Check sheet for the modelled part. Datum: model origin and axes. Units: mm. A direction names the side the tool comes from. Coordinates: 2 decimals unless noted, no trailing zeros. Loops run counter-clockwise (first coordinate to the right, second up) from the corner with the lowest first, then second, coordinate; pieces in that order, holes last.
from build123d import *

# Parameters (mm, degrees)
SKETCH1_W           = 25.4
SKETCH1_H           = 25.4
BOSS_EXTRUDE1_DEPTH = 5.91
BOSS_EXTRUDE2_DEPTH = 25.4
BOSS_EXTRUDE3_DEPTH = 25.4
BOSS_EXTRUDE4_DEPTH = 25.4
FILLET2_R           = 1


with BuildPart() as part:
    # Sketch1 → Boss-Extrude1 (new body)
    with BuildSketch(Plane(origin=(0, 0, 0), x_dir=(1, 0, 0), z_dir=(0, 1, 0))):
        Rectangle(SKETCH1_W, SKETCH1_H)
    extrude(amount=BOSS_EXTRUDE1_DEPTH)

    # Sketch2 → Boss-Extrude2 (add)
    with BuildSketch(Plane.XY.offset(12.7)):
        Polygon((-3, 0), (3, 0), (3, 2.5), (6, 2.5), (6, 4.5), (4.585786438, 5.914213562), (-4.585786438, 5.914213562), (-6, 4.5), (-6, 2.5), (-3, 2.5), align=None)
    extrude(amount=BOSS_EXTRUDE2_DEPTH)

    # Sketch3 → Boss-Extrude3 (add)
    with BuildSketch(Plane.ZY.offset(12.7)):
        Polygon((-3, 0), (3, 0), (3, 2.5), (6, 2.5), (6, 4.5), (4.585786438, 5.914213562), (-4.585786438, 5.914213562), (-6, 4.5), (-6, 2.5), (-3, 2.5), align=None)
    extrude(amount=BOSS_EXTRUDE3_DEPTH)

    # Sketch5 → Boss-Extrude4 (add)
    with BuildSketch(Plane(origin=(0, 5.91, 0), x_dir=(1, 0, 0), z_dir=(0, 1, 0))):
        Polygon((3, 12.7), (-3, 12.7), (-3, 10.2), (-6, 10.2), (-6, 8.2), (-4.585786438, 6.785786438), (4.585786438, 6.785786438), (6, 8.2), (6, 10.2), (3, 10.2), align=None)
        Polygon((12.7, -3), (12.7, 3), (10.2, 3), (10.2, 6), (8.2, 6), (6.785786438, 4.585786438), (6.785786438, -4.585786438), (8.2, -6), (10.2, -6), (10.2, -3), align=None)
    extrude(amount=BOSS_EXTRUDE4_DEPTH)

    # Fillet2
    fillet2_edges = [part.edges().sort_by_distance(p)[0] for p in [
        (6.785786438, 5.91, 0),
        (7.492893219, 5.91, 5.292893219),
        (9.2, 5.91, 6),
        (10.2, 5.91, 4.5),
        (11.45, 5.91, 3),
        (12.7, 18.61, 3),
        (-12.7, 5.91, -8.645),
        (7.85, 0, 12.7),
        (8.645, 5.91, 12.7),
        (-8.645, 5.91, 12.7),
        (3, 0, 25.4),
        (-3, 0, 25.4),
        (0, 0, 38.1),
        (-12.7, 0, 7.85),
        (-12.7, 5.91, 8.645),
        (-25.4, 0, 3),
        (12.7, 5.91, 7.85),
        (-7.85, 0, 12.7),
        (-12.7, 0, -7.85),
        (-25.4, 0, -3),
        (-38.1, 0, 0),
        (0, 0, -12.7),
        (12.7, 0, 0),
        (12.7, 5.91, -7.85),
        (-7.85, 5.91, -12.7),
        (-3, 5.91, -11.45),
        (-3, 18.61, -12.7),
        (-4.5, 5.91, -10.2),
        (-6, 5.91, -9.2),
        (-5.292893219, 5.91, -7.492893219),
        (0, 5.91, -6.785786438),
        (5.292893219, 5.91, -7.492893219),
        (6, 5.91, -9.2),
        (4.5, 5.91, -10.2),
        (3, 5.91, -11.45),
        (3, 18.61, -12.7),
        (7.85, 5.91, -12.7),
        (11.45, 5.91, -3),
        (12.7, 18.61, -3),
        (10.2, 5.91, -4.5),
        (9.2, 5.91, -6),
        (7.492893219, 5.91, -5.292893219),
    ]]
    fillet(fillet2_edges, radius=FILLET2_R)


solid = part.part
(1) Set-up check for faces 1 (the face through (5, 19, -10.2)), 2 (the face through (0, 5.914, 25)), 3 (the face through (6.786, 19, 0)): record each of +Z, -Z, +X, -X, +Y, -Y from which the full face is reachable in a straight line by a thin tool's end or side.
(2) Section check B-B, the plane z = 30.5. Enter the section's corners in (x, y).
(3) Section check C-C, the plane x = -9. Enter the section's corners in (y, z).
(4) Scan lines: line 1 along X through (y, z) = (3, -11); line 2 along X through (y, z) = (4, 18); line 3 along Z through (x, y) = (-33, 2). Record each from-to range of solid material in increasing order.
(5) Gauge pin test, flat ends, axial feed: P1, Ø3.5, axis at x = -4, z = 22, coming from the -Y side; P2, Ø10, axis at x = -21, z = 2, coming from the +Y side; P3, Ø1.6, axis at x = 9.5, y = 24, coming from the +Z side; P4, Ø3, axis at y = 3.5, z = -7, coming from the -X side. Record the tip position at first contact, or that the pin passes through.
(6) Section check A-A, the plane y = 18. Enter the section's corners in (x, z), plus the area to 3 significant figures.
(7) Section check D-D, the plane x = 9.5. Enter the section's corners in (y, z).
Determined:
1. face 1: -Z, +X, +Y
1. face 2: +Z, +X, -X, +Y
1. face 3: +Z, -Z, -X, +Y
2. outline: (-6, 2.5) - (-3, 2.5) - (-3, 1) arc R1 ccw to (-2, 0) - (2, 0) arc R1 ccw to (3, 1) - (3, 2.5) - (6, 2.5) - (6, 4.5) - (4.59, 5.91) - (-4.59, 5.91) - (-6, 4.5) - close
3. outline: (0, -11.7) arc R1 ccw to (1, -12.7) - (4.91, -12.7) arc R1 ccw to (5.91, -11.7) - (5.91, 11.7) arc R1 ccw to (4.91, 12.7) - (1, 12.7) arc R1 ccw to (0, 11.7) - close
4. line 1: x = -12.7 to 12.7
4. line 2: x = -6 to 6
4. line 3: z = -3 to 3
5. P1: stops at y = 0.03
5. P2: stops at y = 5.91
5. P3: stops at z = 6
5. P4: stops at x = -38.1
6. outline: (-6, -10.2) - (-3, -10.2) - (-3, -11.7) arc R1 ccw to (-2, -12.7) - (2, -12.7) arc R1 ccw to (3, -11.7) - (3, -10.2) - (6, -10.2) - (6, -8.2) - (4.59, -6.79) - (-4.59, -6.79) - (-6, -8.2) - close; (6.79, -4.59) - (8.2, -6) - (10.2, -6) - (10.2, -3) - (11.7, -3) arc R1 ccw to (12.7, -2) - (12.7, 2) arc R1 ccw to (11.7, 3) - (10.2, 3) - (10.2, 6) - (8.2, 6) - (6.79, 4.59) - close
6. area: 107 mm2
7. outline: (0, -11.7) arc R1 ccw to (1, -12.7) - (4.91, -12.7) arc R1 ccw to (5.91, -11.7) - (5.91, -7) arc R1 cw to (6.91, -6) - (31.31, -6) - (31.31, 6) - (6.91, 6) arc R1 cw to (5.91, 7) - (5.91, 11.7) arc R1 ccw to (4.91, 12.7) - (1, 12.7) arc R1 ccw to (0, 11.7) - close
